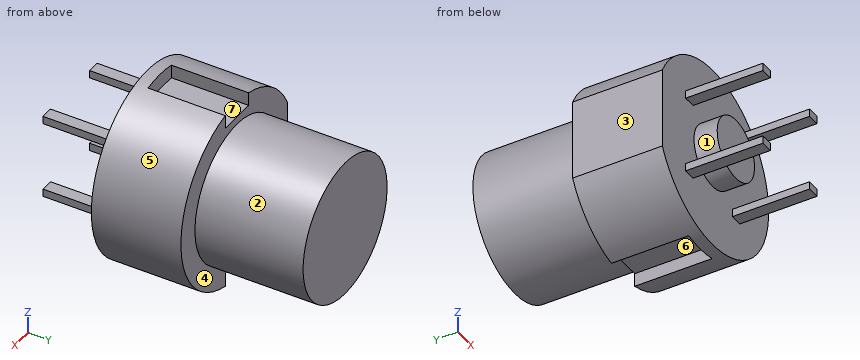
```python
from build123d import *

# Parameters (mm, degrees)
SKETCH2_W      = 0.8
SKETCH2_H      = 0.5
LEGS_DEPTH     = 5
SKETCH3_W      = 4.6
SKETCH3_H      = 13.743650636
EXTRUDE3_DEPTH = 20.719026345
SKETCH4_W      = 2.5
SKETCH4_H      = 2
EXTRUDE4_DEPTH = 5


with BuildPart() as part:
    # Sketch1 → Revolve1 (revolve)
    with BuildSketch(Plane.XY, mode=Mode.PRIVATE) as revolve1_sk:
        Polygon((0, 0), (2, 0), (2, 1.5), (6, 1.5), (6, 7.3), (4.5, 7.3), (4.5, 14.3), (0, 14.3), align=None)
    revolve(revolve1_sk.sketch.rotate(Axis((0, 33.182896664, 0), (0, -1, 0)), 90), axis=Axis((0, 33.182896664, 0), (0, -1, 0)))

    # Sketch2 → Legs (add)
    with BuildSketch(Plane.XZ.offset(-1.5)):
        with Locations((-2.5, 2.5)):
            Rectangle(SKETCH2_W, SKETCH2_H)
        with Locations((2.5, 2.5)):
            Rectangle(SKETCH2_W, SKETCH2_H)
        with Locations((2.5, -2.5)):
            Rectangle(SKETCH2_W, SKETCH2_H)
        with Locations((-2.5, -2.5)):
            Rectangle(SKETCH2_W, SKETCH2_H)
    extrude(amount=LEGS_DEPTH)

    # Sketch3 → Extrude3 (cut, through all)
    with BuildSketch(Plane(origin=(0, 14.3, 0), x_dir=(1, 0, 0), z_dir=(0, 1, 0))):
        with Locations((-7.7, -0.438016034)):
            Rectangle(SKETCH3_W, SKETCH3_H)
    extrude(amount=-EXTRUDE3_DEPTH, mode=Mode.SUBTRACT)

    # Sketch4 → Extrude4 (cut)
    with BuildSketch(Plane(origin=(0, 7.3, 0), x_dir=(1, 0, 0), z_dir=(0, 1, 0))):
        with Locations((0, 6)):
            Rectangle(SKETCH4_W, SKETCH4_H)
        with Locations((0, -6)):
            Rectangle(SKETCH4_W, SKETCH4_H)
    extrude(amount=-EXTRUDE4_DEPTH, mode=Mode.SUBTRACT)


solid = part.part
```
Read the model definition and answer for the solid it produces. Units are mm, in the model's axes. Face numbers are marked on the shaded views. A direction names the side the tool comes from. Give positions to 0.01 mm unless a question says otherwise; leave off trailing zeros. Order: outer loops, then holes, each group sorted by start corner. A loop starts at its lowest first (then second) coordinate and runs counter-clockwise, first axis right, second up. Notation, with made-up numbers: (36, 65.25) -> (40, 65.25) arc R21 cw to (40, 78.25) -> close; hole circle Ø11 at (44.5, -8). An arc over 180 degrees is marked (long way). One line per item, written item: value. Start each with the question number.
(1) The part is cut by section A-A (z = 0). Determine the outline of the cut face in (x, y).
(2) For a pull along X with two mould halves and no side action, classify the marked faces 4, 5, 6 and 7 as released by +X, released by -X, zero draft, split by the parting line, or undercut.
(3) The part is cut by section D-D (z = 3.5). Determine the outline of the cut face in (x, y).
(4) The part is cut by section C-C (x = 0). Determine the outline of the cut face in (y, z), and give its area (3 significant figures).
(5) A tool of negligible diameter and unlimited length cuts with its end or side. For the marked faces 1, 2 and 3, from which of +Z, -Z, +X, -X, +Y, -Y can it reach the whole face along a straight path? Write none if from no direction.
(6) Flat-ended cylindrical pins translate along their axes: P1, Ø3, axis at x = 0, z = 0, coming from the -Y side; P2, Ø0.9, axis at x = -2.5, y = -1.5, coming from the -Z side; P3, Ø0.7, axis at y = 5, z = -5.5, coming from the -X side. Find the tip coordinate at first contact, or state that the pin passes through.
(7) The part is cut by section B-B (y = 4). Determine the outline of the cut face in (x, z), and give its area (3 significant figures).
(8) Straight lines are drawn through the part: L1, parallel to Y at x = -2.5, z = 1; L2, parallel to Y at x = -1.25, z = 0.5; L3, parallel to X at y = 2.5, z = -1.25. For each, find the intervals that lie inside material, in ascending order.
Taken from the geometry:
1. outline: (-5.4, 1.5) -> (-2, 1.5) -> (-2, 0) -> (2, 0) -> (2, 1.5) -> (6, 1.5) -> (6, 7.3) -> (4.5, 7.3) -> (4.5, 14.3) -> (-4.5, 14.3) -> (-4.5, 7.3) -> (-5.4, 7.3) -> close
2. face 4: zero draft
2. face 5: split by the parting line
2. face 6: undercut
2. face 7: undercut
3. outline: (-4.87, 1.5) -> (4.87, 1.5) -> (4.87, 7.3) -> (2.83, 7.3) -> (2.83, 14.3) -> (-2.83, 14.3) -> (-2.83, 7.3) -> (-4.87, 7.3) -> close
4. outline: (0, -2) -> (1.5, -2) -> (1.5, -6) -> (2.3, -6) -> (2.3, -5) -> (7.3, -5) -> (7.3, -4.5) -> (14.3, -4.5) -> (14.3, 4.5) -> (7.3, 4.5) -> (7.3, 5) -> (2.3, 5) -> (2.3, 6) -> (1.5, 6) -> (1.5, 2) -> (0, 2) -> close
4. area: 129 mm^2
5. face 1: -Y
5. face 2: +Y
5. face 3: +Z, -Z, -X, +Y, -Y
6. P1: y = 0
6. P2: z = -2.75
6. P3: x = -3.08
7. outline: (-5.4, -2.62) arc R6 ccw to (-1.25, -5.87) -> (-1.25, -5) -> (1.25, -5) -> (1.25, -5.87) arc R6 ccw to (1.25, 5.87) -> (1.25, 5) -> (-1.25, 5) -> (-1.25, 5.87) arc R6 ccw to (-5.4, 2.62) -> close
7. area: 106 mm^2
8. L1: 1.5 to 14.3
8. L2: 0 to 14.3
8. L3: -5.4 to 5.87
